Geometry check sheet. Reference: the model listing, model coordinates, mm. Round coordinates to 2 decimals unless told otherwise and drop trailing zeros. Write each loop counter-clockwise with the first axis right and the second up, starting at its lowest first coordinate (ties: lowest second). Pieces come first, ordered by that corner, then holes. Notation, with made-up numbers: (1, -15) -> (43, -15) arc R29 cw to (43, 9) -> close; hole circle Ø3 at (48.5, 28.25). An arc over 180 degrees is marked (long way). One line per question, with ' | ' between items.
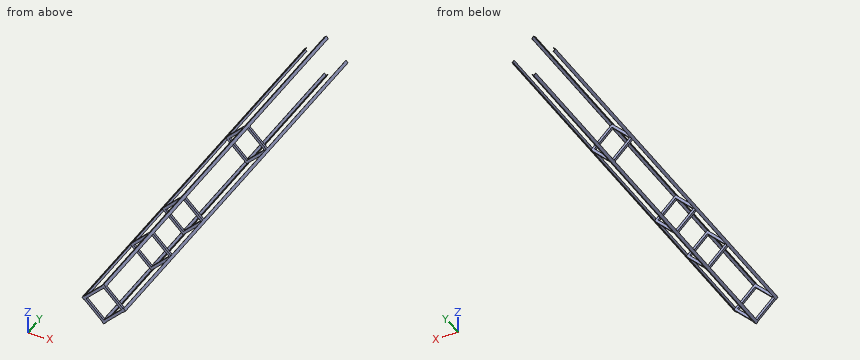
```python
from build123d import *

# Parameters (mm, degrees)
BOSS_EXTRUDE6_DEPTH   = 1778
BOSS_EXTRUDE6_2_DEPTH = 1778
BOSS_EXTRUDE6_3_DEPTH = 1778
BOSS_EXTRUDE6_4_DEPTH = 1778
SKETCH11_W            = 11.1125
SKETCH11_H            = 9.525
BOSS_EXTRUDE11_DEPTH  = 129.12986
SKETCH13_W            = 11.1125
SKETCH13_H            = 9.525
BOSS_EXTRUDE13_DEPTH  = 118.01736
SKETCH14_W            = 11.1125
SKETCH14_H            = 9.525
BOSS_EXTRUDE14_DEPTH  = 119.60486
SKETCH15_W            = 11.1125
SKETCH15_H            = 9.525
BOSS_EXTRUDE15_DEPTH  = 106.90486
LPATTERN1_COUNT       = 2
LPATTERN1_PITCH       = 381
LPATTERN2_COUNT       = 2
LPATTERN2_PITCH       = 635
LPATTERN3_COUNT       = 2
LPATTERN3_PITCH       = 1143
SKETCH16_W            = 12.7
SKETCH16_H            = 12.7
BOSS_EXTRUDE16_DEPTH  = 0.0254
SKETCH17_W            = 12.7
SKETCH17_H            = 12.7
BOSS_EXTRUDE17_DEPTH  = 0.0254
SKETCH18_W            = 1.5875
SKETCH18_H            = 12.7
BOSS_EXTRUDE18_DEPTH  = 0.0254
SKETCH19_W            = 1.5875
SKETCH19_H            = 12.7
BOSS_EXTRUDE19_DEPTH  = 0.0254


with BuildPart() as part:
    # Sketch2 → Boss-Extrude6 (new body)
    with BuildSketch(Plane(origin=(0, 0, 0), x_dir=(1, 0, 0), z_dir=(0, 1, 0))):
        Polygon((0, 93.553663338), (-8.980256121, 84.573407217), (-7.857724106, 83.450875201), (0, 91.308599307), (7.857724106, 83.450875201), (8.980256121, 84.573407217), align=None)
    extrude(amount=BOSS_EXTRUDE6_DEPTH)



with BuildPart() as body_2:
    # Sketch2 → Boss-Extrude6 2 (new body)
    with BuildSketch(Plane(origin=(0, 0, 0), x_dir=(1, 0, 0), z_dir=(0, 1, 0))):
        Polygon((93.553663338, 0), (84.573407217, 8.980256121), (83.450875201, 7.857724106), (91.308599307, 0), (83.450875201, -7.857724106), (84.573407217, -8.980256121), align=None)
    extrude(amount=BOSS_EXTRUDE6_2_DEPTH)



with BuildPart() as body_3:
    # Sketch2 → Boss-Extrude6 3 (new body)
    with BuildSketch(Plane(origin=(0, 0, 0), x_dir=(1, 0, 0), z_dir=(0, 1, 0))):
        Polygon((0, -93.553663338), (8.980256121, -84.573407217), (7.857724106, -83.450875201), (0, -91.308599307), (-7.857724106, -83.450875201), (-8.980256121, -84.573407217), align=None)
    extrude(amount=BOSS_EXTRUDE6_3_DEPTH)



with BuildPart() as body_4:
    # Sketch2 → Boss-Extrude6 4 (new body)
    with BuildSketch(Plane(origin=(0, 0, 0), x_dir=(1, 0, 0), z_dir=(0, 1, 0))):
        Polygon((-93.553663338, 0), (-84.573407217, -8.980256121), (-83.450875201, -7.857724106), (-91.308599307, 0), (-83.450875201, 7.857724106), (-84.573407217, 8.980256121), align=None)
    extrude(amount=BOSS_EXTRUDE6_4_DEPTH)


with BuildPart() as body_3_1:
    add(body_3.part)

    add(body_4.part)  # Boss-Extrude11 merges body 4
    # Sketch11 → Boss-Extrude11 (add)
    with BuildSketch(Plane(origin=(-45.654299654, 0, -45.654299654), x_dir=(0.707106781, 0, -0.707106781), z_dir=(0.707106781, 0, 0.707106781))):
        with Locations((-59.008679751, 4.7625)):
            Rectangle(SKETCH11_W, SKETCH11_H)
    boss_extrude11 = extrude(amount=BOSS_EXTRUDE11_DEPTH)


with BuildPart() as body_2_1:
    add(body_2.part)

    add(body_3_1.part)  # Boss-Extrude13 merges body 3
    # Sketch13 → Boss-Extrude13 (add)
    with BuildSketch(Plane(origin=(-37.796575548, 0, 37.796575548), x_dir=(-0.707106781, 0, -0.707106781), z_dir=(0.707106781, 0, -0.707106781))):
        with Locations((-59.008679751, 4.7625)):
            Rectangle(SKETCH13_W, SKETCH13_H)
    boss_extrude13 = extrude(amount=BOSS_EXTRUDE13_DEPTH)


with BuildPart() as part_1:
    add(part.part)

    add(body_2_1.part)  # Boss-Extrude14 merges body 2
    # Sketch14 → Boss-Extrude14 (add)
    with BuildSketch(Plane(origin=(37.796575548, 0, 37.796575548), x_dir=(-0.707106781, 0, 0.707106781), z_dir=(-0.707106781, 0, -0.707106781))):
        with Locations((-59.008679751, 4.7625)):
            Rectangle(SKETCH14_W, SKETCH14_H)
    boss_extrude14 = extrude(amount=BOSS_EXTRUDE14_DEPTH)

    # Sketch15 → Boss-Extrude15 (add)
    with BuildSketch(Plane(origin=(37.796575548, 0, -37.796575548), x_dir=(0.707106781, 0, 0.707106781), z_dir=(-0.707106781, 0, 0.707106781))):
        with Locations((-59.008679751, 4.7625)):
            Rectangle(SKETCH15_W, SKETCH15_H)
    boss_extrude15 = extrude(amount=BOSS_EXTRUDE15_DEPTH)

    # LPattern1: Boss-Extrude11, Boss-Extrude13, Boss-Extrude14, Boss-Extrude15 ×2
    with Locations(*[(0, i * LPATTERN1_PITCH, 0) for i in range(1, LPATTERN1_COUNT)]):
        add(boss_extrude11)
        add(boss_extrude13)
        add(boss_extrude14)
        add(boss_extrude15)

    # LPattern2: Boss-Extrude11, Boss-Extrude13, Boss-Extrude14, Boss-Extrude15 ×2
    with Locations(*[(0, i * LPATTERN2_PITCH, 0) for i in range(1, LPATTERN2_COUNT)]):
        add(boss_extrude11)
        add(boss_extrude13)
        add(boss_extrude14)
        add(boss_extrude15)

    # LPattern3: Boss-Extrude11, Boss-Extrude13, Boss-Extrude14, Boss-Extrude15 ×2
    with Locations(*[(0, i * LPATTERN3_PITCH, 0) for i in range(1, LPATTERN3_COUNT)]):
        add(boss_extrude11)
        add(boss_extrude13)
        add(boss_extrude14)
        add(boss_extrude15)

    # Sketch16 → Boss-Extrude16 (add)
    with BuildSketch(Plane(origin=(-46.776831669, 0, 46.776831669), x_dir=(0.707106781, 0, 0.707106781), z_dir=(-0.707106781, 0, 0.707106781))):
        with Locations((-59.802429751, 1771.65)):
            Rectangle(SKETCH16_W, SKETCH16_H)
    extrude(amount=BOSS_EXTRUDE16_DEPTH)

    # Sketch17 → Boss-Extrude17 (add)
    with BuildSketch(Plane(origin=(-46.776831669, 0, 46.776831669), x_dir=(0.707106781, 0, 0.707106781), z_dir=(-0.707106781, 0, 0.707106781))):
        with Locations((59.802429751, 1771.65)):
            Rectangle(SKETCH17_W, SKETCH17_H)
    extrude(amount=BOSS_EXTRUDE17_DEPTH)

    # Sketch18 → Boss-Extrude18 (add)
    with BuildSketch(Plane(origin=(37.796575548, 0, -37.796575548), x_dir=(0.707106781, 0, 0.707106781), z_dir=(-0.707106781, 0, 0.707106781))):
        with Locations((-65.358679751, 1771.65)):
            Rectangle(SKETCH18_W, SKETCH18_H)
    extrude(amount=BOSS_EXTRUDE18_DEPTH)

    # Sketch19 → Boss-Extrude19 (add)
    with BuildSketch(Plane(origin=(37.796575548, 0, -37.796575548), x_dir=(0.707106781, 0, 0.707106781), z_dir=(-0.707106781, 0, 0.707106781))):
        with Locations((65.358679751, 1771.65)):
            Rectangle(SKETCH19_W, SKETCH19_H)
    extrude(amount=BOSS_EXTRUDE19_DEPTH)


solid = part_1.part
```
(1) Sectioned sample at B-B on z = -47.5. Count the separate pieces of the cut face and the enclosed holes in it, then the cut area to 3 significant figures.
Resolved:
separate pieces: 8 | enclosed holes: 0 | area: 1,200 mm2
(2) Sectioned sample at A-A on y = 439.5. Record the cut outline in (x, z), then the cut area to 3 significant figures.
Resolved:
outline: (-93.55, 0) -> (-84.57, -8.98) -> (-83.45, -7.86) -> (-91.31, 0) -> (-83.45, 7.86) -> (-84.57, 8.98) -> close; (-8.98, -84.57) -> (0, -93.55) -> (8.98, -84.57) -> (7.86, -83.45) -> (0, -91.31) -> (-7.86, -83.45) -> close; (-8.98, 84.57) -> (-7.86, 83.45) -> (0, 91.31) -> (7.86, 83.45) -> (8.98, 84.57) -> (0, 93.55) -> close; (83.45, -7.86) -> (84.57, -8.98) -> (93.55, 0) -> (84.57, 8.98) -> (83.45, 7.86) -> (91.31, 0) -> close | area: 151 mm2
(3) Go/stop test with a flat-tipped pin: pin 1 (3 mm diameter, centred on x = -16, z = -74, fed in from +Y) (3 decimals). Record where the tip stops, or that it passes through.
Resolved:
pin 1: stops at y = 1152.525
(4) Material ranges on line 1 (Y direction, x = -57, z = 33) (3 decimals); line 2 (X direction, y = 1566, z = 7), recorded low to high.
Resolved:
line 1: y = 0 to 9.525, 381 to 390.525, 635 to 644.525, 1143 to 1152.525 | line 2: x = -86.55 to -84.31, 84.31 to 86.55
